Autodesk Inventor part; units mm, degrees
ref_plane "YZ Plane" through (0, 0, 0) normal (1, 0, 0) x (0, 1, 0)
ref_plane "XZ Plane" through (0, 0, 0) normal (0, 1, 0) x (-1, 0, 0)
ref_plane "XY Plane" through (0, 0, 0) normal (0, 0, 1) x (1, 0, 0)
sketch "Sketch1" plane through (0, 0, 0) normal (0, 0, 1) x (1, 0, 0)
  circle A0 centre (0, 0) radius 30
  dimension "d0" = 60
extrude "Extrusion1" add sketch "Sketch1" along normal blind 10
sketch "Sketch2" plane through (0, 0, 10) normal (0, 0, 1) x (1, 0, 0)
  circle A0 centre (6.2371, -22.9812) radius 1.9939
  circle A1 centre (23.0208, -6.0891) radius 1.9939
  circle A2 centre (-23.0208, 6.0891) radius 1.9939
  circle A3 centre (-16.7837, -16.8921) radius 1.9939
  circle A4 centre (-6.2371, 22.9812) radius 1.9939
  circle A5 centre (16.7837, 16.8921) radius 1.9939
  circle A6 centre (0, 0) radius 14.2875 construction
  point P0 (0, 0)
extrude "Extrusion2" cut sketch "Sketch2" against normal through all
sketch "Sketch3" plane through (0, 0, 0) normal (0, 0, -1) x (-1, 0, 0)
  circle A0 centre (-13.511, -4.1777) radius 2
  circle A1 centre (-4.1777, 13.511) radius 2
  circle A2 centre (4.1777, -13.511) radius 2
  circle A3 centre (13.511, 4.1777) radius 2
  circle A4 centre (4.1777, -13.511) radius 2
  point P0 (0, 0)
extrude "Extrusion3" cut sketch "Sketch3" against normal through all
sketch "Sketch4" plane through (0, 0, 0) normal (0, 0, -1) x (-1, 0, 0)
  circle A0 centre (0, 0) radius 4 construction
  circle A1 centre (-4.1777, 13.511) radius 2
  circle A2 centre (13.511, 4.1777) radius 2
  circle A3 centre (-13.511, -4.1777) radius 2
  circle A4 centre (4.1777, -13.511) radius 2
  circle A5 centre (-6.2371, -22.9812) radius 1.9939
  circle A6 centre (6.2371, 22.9812) radius 1.9939
  circle A7 centre (-23.0208, -6.0891) radius 1.9939
  circle A8 centre (16.7837, -16.8921) radius 1.9939
  circle A9 centre (23.0208, 6.0891) radius 1.9939
  circle A10 centre (-16.7837, 16.8921) radius 1.9939
  circle A11 centre (0, 0) radius 30
  circle A12 centre (0, 0) radius 4.25
  dimension "d7" = 8.5
extrude "Extrusion4" cut sketch "Sketch4" against normal through all contours A12
sketch "Sketch5" plane through (0, 0, 0) normal (0, 0, -1) x (-1, 0, 0)
  circle A0 centre (0, 0) radius 12.25 construction
  circle A1 centre (0, 0) radius 4.25
  circle A2 centre (0, 0) radius 12
  dimension "d10" = 24
properties part number "LegHub"
CAD build for the part. Positions are in the model's coordinates, mm. Coordinates: 2 decimals unless noted, no trailing zeros. Order: outer loops, then holes, each group sorted by start corner. A loop starts at its lowest first (then second) coordinate and runs counter-clockwise, first axis right, second up. Notation, with made-up numbers: (55.25, 18.25) - (71.25, 18.25) arc R19 cw to (71.25, 30.25) - close; hole circle Ø3 at (88, 11.25). An arc over 180 degrees is marked (long way). Use a Markdown table: item, result. Add a question column.
(1) Saw through at D-D (x = -20). Give the cut face in (y, z).
(2) Pull direction Y, two halves, no side cores. Call faces 1 (the face through (0, -6, 0)), 2 (the face through (-29.97, -1.32, 4.93)), 3 (the face through (-15, -16, 5)): +Y half, -Y half, draft (parallel to the pull), parting line (faces both ways), or undercut.
(3) Saw through at A-A (x = 0). Give the cut face in (y, z), then the cut area to 3 significant figures.
(4) Drill centre lines: line 1 along X through (y, z) = (-3, 8.75); line 2 along X through (y, z) = (-5.5, 0.5); line 3 along Y through (x, z) = (-15, 8.75). Where is each one in solid material? Low to high. Write a range as [from, to].
(5) Flat gauge pins, fed straight in: pin 1 (1 mm diameter, centred on x = -20, z = 8.5, fed in from -Y); pin 2 (5 mm diameter, centred on x = 16.78, y = 16.89, fed in from -Z); pin 3 (1 mm diameter, centred on x = 14.5, z = 9, fed in from -Y); pin 4 (1 mm diameter, centred on x = -17.5, z = 4.5, fed in from +Y). Where does each tip first touch, or does it go through?
(6) Saw through at C-C (z = 9). Count the separate pieces of the cut face and the enclosed holes in it, then the cut area to 3 significant figures.
Solved:
| question | item | result |
|---|---|---|
| 1 | outline | (-22.36, 0) - (22.36, 0) - (22.36, 10) - (-22.36, 10) - close |
| 2 | face 1 | draft |
| 2 | face 2 | parting line |
| 2 | face 3 | undercut |
| 3 | outline | (-30, 0) - (-4.25, 0) - (-4.25, 10) - (-30, 10) - close; (4.25, 0) - (30, 0) - (30, 10) - (4.25, 10) - close |
| 3 | area | 515 mm² |
| 4 | line 1 | x = [-29.85, -3.01], [3.01, 11.89], [15.13, 29.85] |
| 4 | line 2 | x = [-29.49, 12.01], [15.01, 21.12], [24.93, 29.49] |
| 4 | line 3 | y = [-25.98, -17.78], [-16, 2.84], [5.51, 25.98] |
| 5 | pin 1 | stops at y = -22.8 |
| 5 | pin 2 | stops at z = 0 |
| 5 | pin 3 | stops at y = -26.53 |
| 5 | pin 4 | stops at y = 24.72 |
| 6 | separate pieces | 1 |
| 6 | enclosed holes | 11 |
| 6 | area | 2,650 mm² |
